from build123d import *

# Parameters (mm, degrees)
F2_W     = 0.7
F2_H     = 0.7
F3_DEPTH = 13
F4_DEPTH = 6


with BuildPart() as f1:
    # F0 (on Front) → F1 (revolve)
    with BuildSketch(Plane.XZ):
        Polygon((0, 2), (0, 0), (9.25, 0), (9.25, 9.5), (8.25, 9.5), (8.25, 2.5), (7, 2), align=None)
    revolve(axis=Axis((0, 0, -0.2857148442), (0, 0, -1)))

    # F2 (on Top) → F3 (join)
    with BuildSketch(Plane.XY):
        with BuildLine():
            Line((-2.9795133831, -0.35), (-3.6834087473, -0.35))
            ThreePointArc((-3.6834087473, -0.35), (-2.9989376836, -2.1671116191), (-1.4885221007, -3.3873739026))
            Line((-1.4885221007, -3.3873739026), (-1.4885221007, -4.1405678301))
            ThreePointArc((-1.4885221007, -4.1405678301), (-1.1424042215, -4.2491072703), (-0.7885221007, -4.3287680576))
            Line((-0.7885221007, -4.3287680576), (-0.7885221007, -3.6150010922))
            Line((-0.7885221007, -3.6150010922), (-0.7885221007, -2.8945177313))
            ThreePointArc((-0.7885221007, -2.8945177313), (-2.2733599524, -1.9575072227), (-2.9795133831, -0.35))
        make_face()
        with BuildLine():
            Line((-0.35, 1.85), (-0.35, 2.55))
            Line((-0.35, 2.55), (-2.6809513237, 2.55))
            ThreePointArc((-2.6809513237, 2.55), (-3.366937745, 1.5341871534), (-3.6834087473, 0.35))
            Line((-3.6834087473, 0.35), (-2.9795133831, 0.35))
            ThreePointArc((-2.9795133831, 0.35), (-2.7739084983, 1.1425548752), (-2.3616731357, 1.85))
            Line((-2.3616731357, 1.85), (-0.35, 1.85))
        make_face()
        with BuildLine():
            Line((2.6809513237, 2.55), (0.35, 2.55))
            Line((0.35, 2.55), (0.35, 1.85))
            Line((0.35, 1.85), (2.3616731357, 1.85))
            ThreePointArc((2.3616731357, 1.85), (2.7739084983, 1.1425548752), (2.9795133831, 0.35))
            Line((2.9795133831, 0.35), (3.6834087473, 0.35))
            ThreePointArc((3.6834087473, 0.35), (3.366937745, 1.5341871534), (2.6809513237, 2.55))
        make_face()
        with BuildLine():
            ThreePointArc((3.6834087473, -0.35), (3.7, 0), (3.6834087473, 0.35))
            Line((3.6834087473, 0.35), (2.9795133831, 0.35))
            ThreePointArc((2.9795133831, 0.35), (3, 0), (2.9795133831, -0.35))
            Line((2.9795133831, -0.35), (3.6834087473, -0.35))
        make_face()
        with Locations((0, 2.2)):
            Rectangle(F2_W, F2_H)
        with BuildLine():
            Line((-2.9795133831, 0.35), (-3.6834087473, 0.35))
            ThreePointArc((-3.6834087473, 0.35), (-3.7, 0), (-3.6834087473, -0.35))
            Line((-3.6834087473, -0.35), (-2.9795133831, -0.35))
            ThreePointArc((-2.9795133831, -0.35), (-3, 0), (-2.9795133831, 0.35))
        make_face()
        with BuildLine():
            ThreePointArc((1.4885221007, -3.3873739026), (2.9989376836, -2.1671116191), (3.6834087473, -0.35))
            Line((3.6834087473, -0.35), (2.9795133831, -0.35))
            ThreePointArc((2.9795133831, -0.35), (2.2733599524, -1.9575072227), (0.7885221007, -2.8945177313))
            Line((0.7885221007, -2.8945177313), (0.7885221007, -3.6150010922))
            Line((0.7885221007, -3.6150010922), (0.7885221007, -4.3287680576))
            ThreePointArc((0.7885221007, -4.3287680576), (1.1424042215, -4.2491072703), (1.4885221007, -4.1405678301))
            Line((1.4885221007, -4.1405678301), (1.4885221007, -3.3873739026))
        make_face()
        with BuildLine():
            ThreePointArc((-3.6834087473, -0.35), (-3.7, 0), (-3.6834087473, 0.35))
            Line((-3.6834087473, 0.35), (-4.3860574552, 0.35))
            ThreePointArc((-4.3860574552, 0.35), (-4.4, 0), (-4.3860574552, -0.35))
            Line((-4.3860574552, -0.35), (-3.6834087473, -0.35))
        make_face()
        with BuildLine():
            Line((0.35, 2.55), (0.35, 2.9795133831))
            ThreePointArc((0.35, 2.9795133831), (0, 3), (-0.35, 2.9795133831))
            Line((-0.35, 2.9795133831), (-0.35, 2.55))
            Line((-0.35, 2.55), (0.35, 2.55))
        make_face()
        with BuildLine():
            Line((4.3860574552, 0.35), (3.6834087473, 0.35))
            ThreePointArc((3.6834087473, 0.35), (3.7, 0), (3.6834087473, -0.35))
            Line((3.6834087473, -0.35), (4.3860574552, -0.35))
            ThreePointArc((4.3860574552, -0.35), (4.4, 0), (4.3860574552, 0.35))
        make_face()
    extrude(amount=F3_DEPTH)

    # F2 (on Top) → F4 (join)
    with BuildSketch(Plane.XY):
        with BuildLine():
            Line((0.35, 0.35), (0.35, 1.85))
            Line((0.35, 1.85), (-0.35, 1.85))
            Line((-0.35, 1.85), (-0.35, 0.35))
            Line((-0.35, 0.35), (-2.9795133831, 0.35))
            ThreePointArc((-2.9795133831, 0.35), (-3, 0), (-2.9795133831, -0.35))
            Line((-2.9795133831, -0.35), (-0.35, -0.35))
            Line((-0.35, -0.35), (-0.35, -2.9795133831))
            ThreePointArc((-0.35, -2.9795133831), (-0.5708451705, -2.9451885833), (-0.7885221007, -2.8945177313))
            Line((-0.7885221007, -2.8945177313), (-0.7885221007, -3.6150010922))
            ThreePointArc((-0.7885221007, -3.6150010922), (0, -3.7), (0.7885221007, -3.6150010922))
            Line((0.7885221007, -3.6150010922), (0.7885221007, -2.8945177313))
            ThreePointArc((0.7885221007, -2.8945177313), (0.5708451705, -2.9451885833), (0.35, -2.9795133831))
            Line((0.35, -2.9795133831), (0.35, -0.35))
            Line((0.35, -0.35), (2.9795133831, -0.35))
            ThreePointArc((2.9795133831, -0.35), (3, 0), (2.9795133831, 0.35))
            Line((2.9795133831, 0.35), (0.35, 0.35))
        make_face()
    extrude(amount=F4_DEPTH)


solid = f1.part
Input: part model. Units: mm. Frame: model coordinates. Coordinates: 2 decimals unless noted, no trailing zeros. Order: outer loops, then holes, each group sorted by start corner. A loop starts at its lowest first (then second) coordinate and runs counter-clockwise, first axis right, second up. Notation, with made-up numbers: M 74.25,19 L 115.25,19 A22 ccw 115.25,39 Z; hole C -20,7.25 d5. An arc over 180 degrees is marked long. Answer as CSV lines item,"result".
1. Section A-A (z = 8.5). Return the cut outline in (x, y).
Reported:
outline,"C 0,0 d18.5; M -4.39,-0.35 L -3.68,-0.35 A3.7 ccw -1.49,-3.39 L -1.49,-4.14 A4.4 ccw -0.79,-4.33 L -0.79,-2.89 A3 cw -2.36,1.85 L 2.36,1.85 A3 cw 0.79,-2.89 L 0.79,-4.33 A4.4 ccw 1.49,-4.14 L 1.49,-3.39 A3.7 ccw 3.68,-0.35 L 4.39,-0.35 A4.4 ccw 4.39,0.35 L 3.68,0.35 A3.7 ccw 2.68,2.55 L 0.35,2.55 L 0.35,2.98 A3 ccw -0.35,2.98 L -0.35,2.55 L -2.68,2.55 A3.7 ccw -3.68,0.35 L -4.39,0.35 A4.4 ccw Z; hole C 0,0 d16.5"
2. Section B-B (x = 0). Return the cut outline in (y, z).
Reported:
outline,"M -9.25,0 L 9.25,0 L 9.25,9.5 L 8.25,9.5 L 8.25,2.5 L 7,2 L 3,2 L 3,13 L 1.85,13 L 1.85,6 L -3.7,6 L -3.7,2 L -7,2 L -8.25,2.5 L -8.25,9.5 L -9.25,9.5 Z"
3. Pull-direction query (Y, two-part tool) for faces 1 (the flat face through (-0.35, 1, 4)), 2 (the cylindrical face through (-2.01, 9.03, 4.82)), 3 (the flat face through (0, 0, 0)); classes: released by +Y, released by -Y, zero draft, split by the parting line, or undercut.
Reported:
face 1,"undercut"
face 2,"split by the parting line"
face 3,"zero draft"
4. Section C-C (y = 0). Return the cut outline in (x, z), then the cut area to 3 significant figures.
Reported:
outline,"M -9.25,0 L 9.25,0 L 9.25,9.5 L 8.25,9.5 L 8.25,2.5 L 7,2 L 4.4,2 L 4.4,13 L 3,13 L 3,6 L -3,6 L -3,13 L -4.4,13 L -4.4,2 L -7,2 L -8.25,2.5 L -8.25,9.5 L -9.25,9.5 Z"
area,"107 mm2"
5. Material intervals for line 1 (Y direction, x = 0, z = 6.75); line 2 (Y direction, x = 0, z = 5.25); line 3 (X direction, y = -2.5, z = 4.25), sorted ascending. Write a range as from..to.
Reported:
line 1,"-9.25..-8.25, 1.85..3, 8.25..9.25"
line 2,"-9.25..-8.25, -3.7..3, 8.25..9.25"
line 3,"-8.91..-7.86, -2.73..-1.66, -0.35..0.35, 1.66..2.73, 7.86..8.91"
6. First-contact query: P1, Ø0.8, axis at x = -2.5, z = 4, coming from the +Y side; P2, Ø0.8, axis at x = 2, y = 1, coming from the +Z side; P3, Ø0.8, axis at x = 4, z = 6, coming from the +Y side; P4, Ø1, axis at x = -7.5, z = 11, coming from the -Y side. Flat tips, straight axial feed; report the tip coordinate or a pass-through.
Reported:
P1,"y = 9.01"
P2,"z = 2"
P3,"y = 8.52"
P4,"through"
